from build123d import *

# Parameters (mm, degrees)
TUBE_SKETCH_R             = 30
TUBE_EXTRUDE_DEPTH        = 120
TUBE_SHELL_T              = -5
SUPPRT_START              = 20
SUPPRT_BAND_EXTRUDE_DEPTH = 20
PIN_SKETCH_R              = 10
PIN_EXTRUDE_DEPTH         = 50
APERTURE_START            = -4
APERTURE_SKETCH_R         = 25
APERTURE_EXTRUDE_DEPTH    = 2
REAR_FILLET_R             = 5


with BuildPart() as part:
    # Tube Sketch → Tube Extrude (new body)
    with BuildSketch(Plane.XY):
        Circle(TUBE_SKETCH_R)
    extrude(amount=-TUBE_EXTRUDE_DEPTH)

    # Tube Shell
    tube_shell_openings = [part.faces().sort_by_distance(p)[0] for p in [
        (0, 0, -120),
    ]]
    offset(amount=TUBE_SHELL_T, openings=tube_shell_openings, kind=Kind.INTERSECTION)

    # Support Band Sketch → Supprt Band Extrude (add)
    with BuildSketch(Plane.XY.offset(-60).offset(SUPPRT_START)):
        with BuildLine():
            Line((-30, 0), (-30, -35))
            Line((-30, -35), (30, -35))
            Line((30, -35), (30, 0))
            ThreePointArc((30, 0), (0, -30), (-30, 0))
        make_face()
    extrude(amount=-SUPPRT_BAND_EXTRUDE_DEPTH)

    # Pin Sketch → Pin Extrude (add)
    with BuildSketch(Plane.XZ.offset(35)):
        with Locations(Location((0, -50, 0), (0, 0, 270))):
            Circle(PIN_SKETCH_R)
    extrude(amount=PIN_EXTRUDE_DEPTH)

    # Aperture Sketch → Aperture Extrude (add)
    with BuildSketch(Plane(origin=(0, 0, -120), x_dir=(-1, 0, 0), z_dir=(0, 0, -1)).offset(APERTURE_START)):
        with Locations(Location((0, 0, 0), (0, 0, 180))):
            Circle(APERTURE_SKETCH_R)
    extrude(amount=APERTURE_EXTRUDE_DEPTH)

    # Rear Fillet
    rear_fillet_edges = [part.edges().sort_by_distance(p)[0] for p in [
        (-30, 0, 0),
    ]]
    fillet(rear_fillet_edges, radius=REAR_FILLET_R)


solid = part.part
The model under review builds one solid part; all positions refer to its coordinate system, in mm. A direction names the side the tool comes from. Round coordinates to 2 decimals unless told otherwise and drop trailing zeros. Write each loop counter-clockwise with the first axis right and the second up, starting at its lowest first coordinate (ties: lowest second). Pieces come first, ordered by that corner, then holes. Notation, with made-up numbers: (54, -8) -> (109, -8) arc R21 ccw to (109, 4) -> close; hole circle Ø10 at (4, 62.5). An arc over 180 degrees is marked (long way). Answer as a JSON object with one key per item and string values.
1. Machinability: for faces 5 (the face through (-0.1, -30.4, -60)), 6 (the face through (-3.905, 29.745, -61.695)), 7 (the face through (-0.1, -30.4, -40)), which of the approach directions +Z, -Z, +X, -X, +Y, -Y give a long, thin tool a straight path to every point of the face, cutting with its end or side? Answer none if there is none.
Results found:
{"face 5": "-Z, -Y", "face 6": "none", "face 7": "+Z, -Y"}
2. We need section B-B on y = -46.5. State the section outline as (x, z) points.
Results found:
{"outline": "circle Ø20 at (0, -50)"}
3. We need section C-C on z = -92. State the section outline as (x, y) points, and give its area (3 significant figures).
Results found:
{"outline": "circle Ø60 at (0, 0); hole circle Ø50 at (0, 0)", "area": "864 mm^2"}
4. Clearance check with flat-ended pins moving along their axes: pin 1 (15 mm diameter, centred on x = 2, y = -11, fed in from +Z); pin 2 (1 mm diameter, centred on y = -31, z = -34, fed in from -X); pin 3 (6 mm diameter, centred on y = 15, z = -14, fed in from +X); pin 4 (4 mm diameter, centred on x = -6, z = -97, fed in from +Y). State where each tip first meets the part, or that it passes through.
Results found:
{"pin 1": "stops at z = 0", "pin 2": "passes through", "pin 3": "stops at x = 27.5", "pin 4": "stops at y = 29.73"}
5. To check wall thickness, follow line 1 along Y through (x, z) = (0, -79); line 2 along Z through (x, y) = (0, 10). State the ranges of each line that lie inside material, in increasing order.
Results found:
{"line 1": "y = -30 to -25, 25 to 30", "line 2": "z = -118 to -116, -5 to 0"}
6. We need section A-A on z = -50. State the section outline as (x, y) points, and give its area (3 significant figures).
Results found:
{"outline": "(-30, -35) -> (-10, -35) -> (-10, -85) -> (10, -85) -> (10, -35) -> (30, -35) -> (30, 0) arc R30 ccw to (-30, 0) -> close; hole circle Ø50 at (0, 0)", "area": "2,550 mm^2"}
7. The part is to be moulded in two halves that separate along X. For faces 1 (the face through (-30, -17, -50)), 2 (the face through (0, 0, -118)), 3 (the face through (0, -60, -40)), 4 (the face through (30, -18, -50)), say which applies: pulls with the +X half, pulls with the -X half, needs draft (parallel to the pull), parting line crosses it, or undercut.
Results found:
{"face 1": "pulls with the -X half", "face 2": "undercut", "face 3": "parting line crosses it", "face 4": "pulls with the +X half"}
